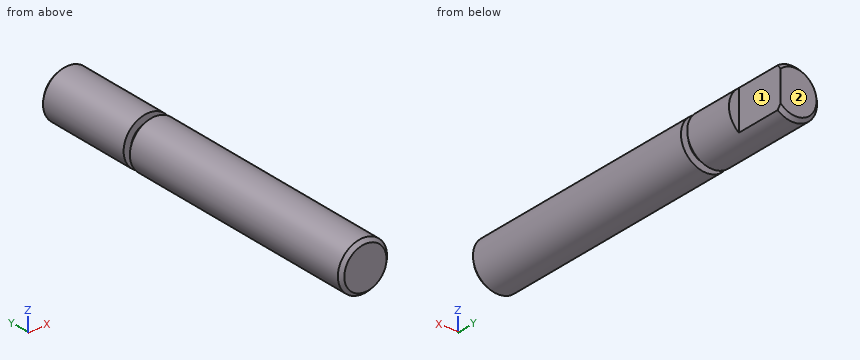
from build123d import *

# Parameters (mm, degrees)
ENL_V_MAT_EXTRU_1_DEPTH      = 73.346388991
ENL_V_MAT_EXTRU_1_DEPTH_BACK = 73.346388991
ESQUISSE2_W                  = 6
ESQUISSE2_H                  = 14


with BuildPart() as part:
    # Esquisse1 → Révolution1 (revolve)
    with BuildSketch(Plane.XY):
        Polygon((0, 0), (-4.292893219, 0), (-5, 0.707106781), (-5, 50.5), (-3.5, 50.5), (-3.5, 52), (-5, 52), (-5, 71.292893219), (-4.292893219, 72), (0, 72), align=None)
    revolve(axis=Axis((0, 72, 0), (0, -1, 0)))

    # Esquisse2 → Enlèv. mat.-Extru.1 (cut, two sides: drawn at the far end of the back side and taken through both)
    with BuildSketch(Plane.XY.offset(-ENL_V_MAT_EXTRU_1_DEPTH_BACK)):
        with Locations((6, 69)):
            Rectangle(ESQUISSE2_W, ESQUISSE2_H)
    extrude(amount=ENL_V_MAT_EXTRU_1_DEPTH + ENL_V_MAT_EXTRU_1_DEPTH_BACK, mode=Mode.SUBTRACT)


solid = part.part
Design review of the part built by this model. Coordinates are the model's own, in mm. Face numbers are marked on the shaded views. A direction names the side the tool comes from. Round coordinates to 2 decimals unless told otherwise and drop trailing zeros. Order: outer loops, then holes, each group sorted by start corner. A loop starts at its lowest first (then second) coordinate and runs counter-clockwise, first axis right, second up.
1) For L1, parallel to Y at x = 4.25, z = 0.5; L2, parallel to Y at x = -0.25, z = 3.75; L3, parallel to Z at x = -3, y = 42, list the stretches that pass through material, from the lowest coordinate up.
The answers:
L1: y = 0 to 50.5, 52 to 62
L2: y = 0 to 50.5, 52 to 72
L3: z = -4 to 4
2) Clearance check with flat-ended pins moving along their axes: pin 1 Ø3 at (y, z) = (38, 4) entering from +X; pin 2 Ø4 at (y, z) = (21, 3) entering from -X; pin 3 Ø0.6 at (x, z) = (4, 1) entering from +Y. State where each tip first meets the part, or that it passes through.
The answers:
pin 1: stops at x = 4.33
pin 2: stops at x = -4.9
pin 3: stops at y = 62
3) Machinability: for the marked faces 1 and 2, which of the approach directions +Z, -Z, +X, -X, +Y, -Y give a long, thin tool a straight path to every point of the face, cutting with its end or side? Answer none if there is none.
The answers:
face 1: +Z, -Z, +X, +Y
face 2: +Z, -Z, +X, -X, +Y
4) Consider section A-A (z = 0). State the section outline as (x, y) points.
The answers:
outline: (-5, 0.71) - (-4.29, 0) - (4.29, 0) - (5, 0.71) - (5, 50.5) - (3.5, 50.5) - (3.5, 52) - (5, 52) - (5, 62) - (3, 62) - (3, 72) - (-4.29, 72) - (-5, 71.29) - (-5, 52) - (-3.5, 52) - (-3.5, 50.5) - (-5, 50.5) - close
5) Consider section B-B (y = 9). State the section outline as (x, z) points, plus the area to 3 significant figures.
The answers:
outline: circle Ø10 at (0, 0)
area: 78.5 mm2
